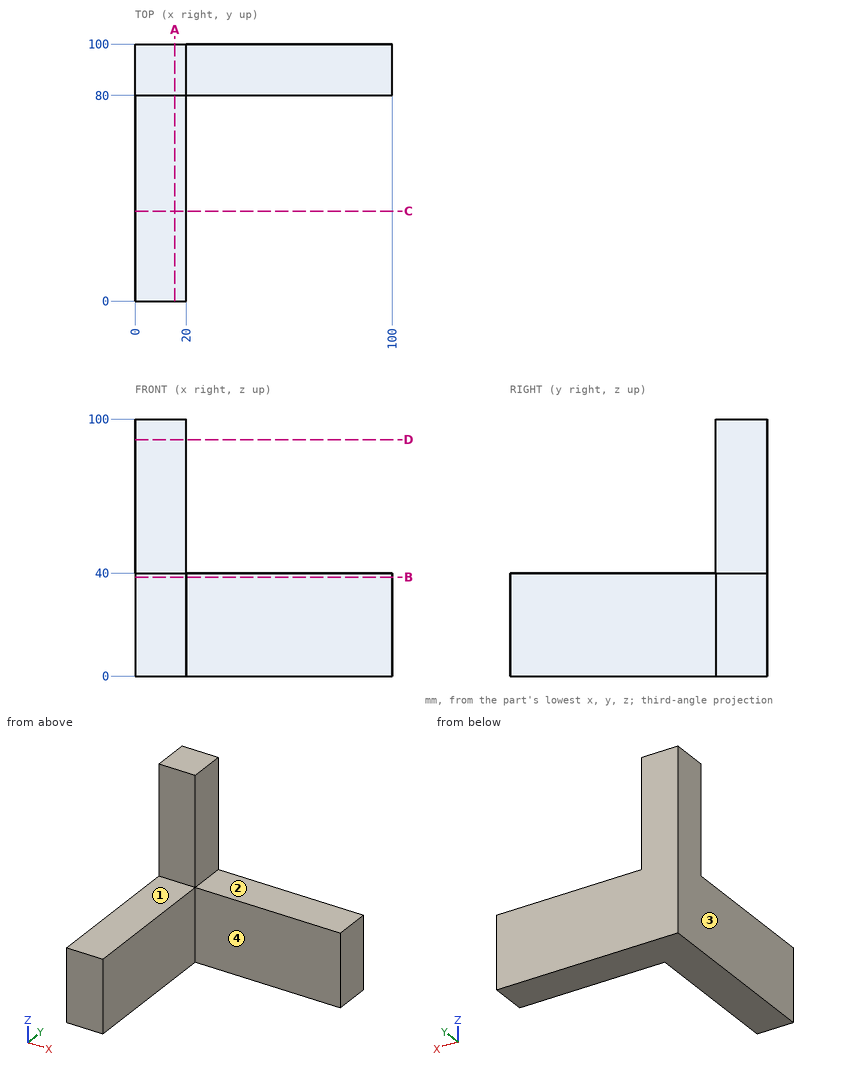
Part print with two shaded views. Sizes in mm from the minimum x, y, z corner. A direction names the side the tool comes from. Round coordinates to 2 decimals unless told otherwise and drop trailing zeros. Order: outer loops, then holes, each group sorted by start corner. A loop starts at its lowest first (then second) coordinate and runs counter-clockwise, first axis right, second up. Notation, with made-up numbers: M 72.5,69.25 L 118.5,69.25 A31 cw 118.5,100.25 Z; hole C 88.5,52 d1. An arc over 180 degrees is marked long. Answer in a Markdown table with one row per item. Add a question column.
Q1. 3-axis set-ups, long thin cutter, end or side, ignore diameter. For the marked faces 1, 2, 3 and 4: which of +Z, -Z, +X, -X, +Y, -Y reach the whole face in a straight line?
Q2. Wall check: L1, parallel to Y at x = 40, z = 21.5; L2, parallel to Z at x = 92.5, y = 95.5; L3, parallel to X at y = 53, z = 17. Give the ranges that are in metal, low to high. Write a range as from..to.
Q3. Cut at B-B on z = 38.5. Give the cut face in (x, y), and give its area (3 significant figures).
Q4. Cut at D-D on z = 92. Give the cut face in (x, y).
Q5. Cut at C-C on y = 35. Give the cut face in (x, z).
Q6. Cut at A-A on x = 15.5. Give the cut face in (y, z), and give its area (3 significant figures).
Q7. Pin check, flat tips, straight feed: pin 1 (22 mm diameter, centred on x = 55, y = 92.5, fed in from +Z); pin 2 (4 mm diameter, centred on y = 70.5, z = 18, fed in from -X); pin 3 (6 mm diameter, centred on y = 92, z = 84, fed in from +X); pin 4 (22 mm diameter, centred on x = 6.5, z = 77.5, fed in from -Y). Stop position of each tip, or through.
Established:
| question | item | result |
|---|---|---|
| 1 | face 1 | +Z, +X, -X, -Y |
| 1 | face 2 | +Z, +X, +Y, -Y |
| 1 | face 3 | +Z, -Z, -X, +Y, -Y |
| 1 | face 4 | +Z, -Z, +X, -Y |
| 2 | L1 | y = 80..100 |
| 2 | L2 | z = 0..40 |
| 2 | L3 | x = 0..20 |
| 3 | outline | M 0,0 L 20,0 L 20,80 L 100,80 L 100,100 L 0,100 Z |
| 3 | area | 3,600 mm2 |
| 4 | outline | M 0,80 L 20,80 L 20,100 L 0,100 Z |
| 5 | outline | M 0,0 L 20,0 L 20,40 L 0,40 Z |
| 6 | outline | M 0,0 L 100,0 L 100,100 L 80,100 L 80,40 L 0,40 Z |
| 6 | area | 5,200 mm2 |
| 7 | pin 1 | stops at z = 40 |
| 7 | pin 2 | stops at x = 0 |
| 7 | pin 3 | stops at x = 20 |
| 7 | pin 4 | stops at y = 80 |
